Verification items for the finished model (mm, model axes). Face numbers are marked on the shaded views. Coordinates: 2 decimals unless noted, no trailing zeros. Order: outer loops, then holes, each group sorted by start corner. A loop starts at its lowest first (then second) coordinate and runs counter-clockwise, first axis right, second up. Notation, with made-up numbers: M 87.25,66.5 L 102.25,66.5 A24 ccw 102.25,88.5 Z; hole C 82,31.5 d10. An arc over 180 degrees is marked long. Answer as a JSON object with one key per item and string values. Group by question number.
(1) Material ranges on line 1 (Y direction, x = 12.7, z = 2.05) (3 decimals); line 2 (Y direction, x = 14.5, z = 1); line 3 (Y direction, x = 38.1, z = 1.75) (3 decimals), recorded low to high.
(2) Cross-section at D-D (x = 12.7). Enter the section's corners in (y, z) (3 decimals).
(3) Gauge pin test, flat ends, axial feed: pin 1 Ø11 at (x, y) = (38.1, 12.7) entering from -Z; pin 2 Ø1 at (x, z) = (55, 1) entering from +Y; pin 3 Ø4 at (x, y) = (63.5, 12.7) entering from -Z. Record the tip position at first contact, or that the pin passes through.
(4) Cross-section at B-B (z = 2.55). Enter the section's corners in (x, y) (3 decimals), plus the area to 3 significant figures.
(5) Mould release check, pull along Z, two halves, no side actions. Record for the marked faces 1 and 2: released by +Z, released by -Z, zero draft, split by the parting line, or undercut.
(6) Cross-section at A-A (x = 38.1). Enter the section's corners in (y, z) (3 decimals), plus the area to 3 significant figures.
Autodesk Fusion 360 part; units mm, degrees
sketch "Sketch1" plane through (0, 0, 0) normal (0, 0, 1) x (1, 0, 0)
  line L0 (0, 0) -> (76.2, 0)
  line L1 (76.2, 0) -> (76.2, 25.4)
  line L2 (76.2, 25.4) -> (25.4, 25.4)
  line L3 (25.4, 25.4) -> (25.4, 76.2)
  line L4 (25.4, 76.2) -> (0, 76.2)
  line L5 (0, 76.2) -> (0, 0)
  line L6 (0, 0) -> (25.4, 25.4) construction
  circle A0 centre (12.7, 12.7) radius 3.425
  circle A1 centre (38.1, 12.7) radius 3.425
  circle A2 centre (63.5, 12.7) radius 3.425
  circle A3 centre (12.7, 38.1) radius 3.425
  circle A4 centre (12.7, 63.5) radius 3.425
  dimension "d1" = 25.4
  dimension "d2" = 25.4
  dimension "d3" = 6.85
  dimension "d4" = 12.7
  dimension "d5" = 25.4
  dimension "d6" = 12.7
  dimension "d7" = 12.7
  dimension "d8" = 12.7
  dimension "d9" = 25.4
extrude "Extrude1" add sketch "Sketch1" along normal blind 3.175
fillet "Fillet1" radius 3 5 edges at (0, 0, 1.5875) (76.2, 0, 1.5875) (76.2, 25.4, 1.5875) (25.4, 76.2, 1.5875) (0, 76.2, 1.5875)
fillet "Fillet1" radius 5 1 edges at (25.4, 25.4, 1.5875)
sketch "DXF" plane through (0, 0, 3.175) normal (0, 0, 1) x (-1, 0, 0)
  arc A0 (-3, -76.2) -> (0, -73.2) centre (-3, -73.2) ccw
  line L0 (0, -73.2) -> (0, -3)
  arc A1 (0, -3) -> (-3, 0) centre (-3, -3) ccw
  line L1 (-3, 0) -> (-73.2, 0)
  arc A2 (-73.2, 0) -> (-76.2, -3) centre (-73.2, -3) ccw
  line L2 (-76.2, -3) -> (-76.2, -22.4)
  arc A3 (-76.2, -22.4) -> (-73.2, -25.4) centre (-73.2, -22.4) ccw
  line L3 (-73.2, -25.4) -> (-30.4, -25.4)
  arc A4 (-25.4, -30.4) -> (-30.4, -25.4) centre (-30.4, -30.4) ccw
  line L4 (-25.4, -30.4) -> (-25.4, -73.2)
  arc A5 (-25.4, -73.2) -> (-22.4, -76.2) centre (-22.4, -73.2) ccw
  line L5 (-22.4, -76.2) -> (-3, -76.2)
  circle A6 centre (-63.5, -12.7) radius 3.425
  circle A7 centre (-12.7, -12.7) radius 3.425
  circle A8 centre (-38.1, -12.7) radius 3.425
  circle A9 centre (-12.7, -63.5) radius 3.425
  circle A10 centre (-12.7, -38.1) radius 3.425
equation "d3 = 0.25 in + 0.5 mm"
equation "d6 = d4"
equation "d7 = d4"
equation "d8 = d7"
equation "d9 = d5"
equation "d10 = ( 1 / 8 ) * 1 in"
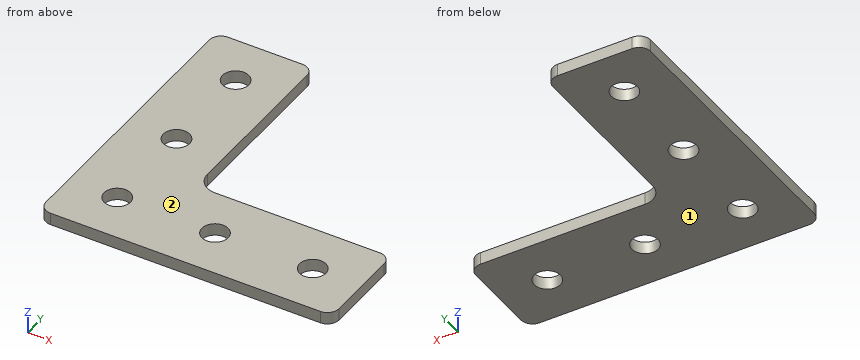
Taken from the geometry:
{
 "1": {"line 1": "y = 0 to 9.275, 16.125 to 34.675, 41.525 to 60.075, 66.925 to 76.2", "line 2": "y = 0 to 9.79, 15.61 to 35.19, 41.01 to 60.59, 66.41 to 76.2", "line 3": "y = 0 to 9.275, 16.125 to 25.4"},
 "2": {"outline": "M 0,0 L 9.275,0 L 9.275,3.175 L 0,3.175 Z; M 16.125,0 L 34.675,0 L 34.675,3.175 L 16.125,3.175 Z; M 41.525,0 L 60.075,0 L 60.075,3.175 L 41.525,3.175 Z; M 66.925,0 L 76.2,0 L 76.2,3.175 L 66.925,3.175 Z"},
 "3": {"pin 1": "stops at z = 0", "pin 2": "stops at y = 25.4", "pin 3": "passes through"},
 "4": {"outline": "M 0,3 A3 ccw 3,0 L 73.2,0 A3 ccw 76.2,3 L 76.2,22.4 A3 ccw 73.2,25.4 L 30.4,25.4 A5 cw 25.4,30.4 L 25.4,73.2 A3 ccw 22.4,76.2 L 3,76.2 A3 ccw 0,73.2 Z; hole C 12.7,12.7 d6.85; hole C 12.7,38.1 d6.85; hole C 12.7,63.5 d6.85; hole C 38.1,12.7 d6.85; hole C 63.5,12.7 d6.85", "area": "3,040 mm²"},
 "5": {"face 1": "released by -Z", "face 2": "released by +Z"},
 "6": {"outline": "M 0,0 L 9.275,0 L 9.275,3.175 L 0,3.175 Z; M 16.125,0 L 25.4,0 L 25.4,3.175 L 16.125,3.175 Z", "area": "58.9 mm²"}
}
